Source: CAD feature listing. Evaluate the final solid. Frame: model axes, mm. A direction names the side the tool comes from. Coordinates: 2 decimals unless noted, no trailing zeros. Loops run counter-clockwise (first coordinate to the right, second up) from the corner with the lowest first, then second, coordinate; pieces in that order, holes last.
Item 1: Reachability of faces 3 (the flat face through (-10, 38, -3)), 4 (the flat face through (35, 0, -2)) from +Z, -Z, +X, -X, +Y, -Y: full face, straight path, thin tool, end or side. Return the list, or none.
Item 2: Section query B-B, the plane z = 6.5. Return the cut outline in (x, y).
Item 3: Section query C-C, the plane y = 0. Return the cut outline in (x, z).
Item 4: Pull-direction query (Z, two-part tool) for faces 1 (the flat face through (-10, -39, -3)), 2 (the cylindrical face through (-3.252, 14.643, 36.949)); classes: +Z half, -Z half, draft (parallel to the pull), parting line (faces both ways), or undercut.
Item 5: Section query A-A, the plane x = 18. Return the cut outline in (y, z).
Item 6: Line query: probe 1 along Z at (x, y) = (-19, 25); probe 2 along Y at (x, z) = (0, 38); probe 3 along Z at (x, y) = (-20.5, -10). Output: solid intervals per line, ascending.
Item 7: Pin query (flat end, axial travel): pin 1 Ø1.5 at (x, z) = (-23.5, 31.5) entering from -Y; pin 2 Ø1.5 at (y, z) = (11, -17.5) entering from +X; pin 3 Ø22.5 at (x, y) = (16, 10) entering from -Z; pin 4 Ø20 at (y, z) = (6, -5) entering from -X. Return the tip coordinate at first contact, or that it passes through.
Item 8: Section query D-D, the plane x = 0. Return the cut outline in (y, z), then the cut area to 3 significant figures.
Autodesk Inventor part; units mm, degrees
ref_plane "YZ Plane" through (0, 0, 0) normal (1, 0, 0) x (0, 1, 0)
ref_plane "XZ Plane" through (0, 0, 0) normal (0, 1, 0) x (-1, 0, 0)
ref_plane "XY Plane" through (0, 0, 0) normal (0, 0, 1) x (1, 0, 0)
sketch "Эскиз1" plane through (0, 0, 0) normal (0, 0, 1) x (1, 0, 0)
  arc A0 (45, 0) -> (-45, 0) centre (0, 0) ccw
  arc A1 (35, 0) -> (-35, 0) centre (0, 0) ccw
  line L0 (-45, 0) -> (-35, 0)
  line L1 (35, 0) -> (45, 0)
  line L2 (-63, 0) -> (63, 0)
  dimension "d0" = 45
  dimension "d1" = 35
revolve "Вращение1" add sketch "Эскиз1" angle 360 about axis through (-10, 0, 0) along (1, 0, 0) contours L1 A1 L0 A0
sketch "Эскиз2" plane through (0, 0, 0) normal (0, 0, 1) x (1, 0, 0)
  circle A0 centre (0, 0) radius 15
  dimension "d3" = 30
extrude "Выдавливание1" cut sketch "Эскиз2" along normal through all
sketch "Эскиз3" plane through (0, 0, 0) normal (0, 1, 0) x (-1, 0, 0)
  line L0 (-35, -15) -> (10, -15)
  line L1 (10, -15) -> (10, 10)
  line L2 (10, 10) -> (-35, 10)
  line L3 (-35, 10) -> (-35, -15)
  point P0 (0, 0)
  dimension "d6" = 10
  dimension "d7" = 45
  dimension "d8" = 10
  dimension "d9" = 25
extrude "Выдавливание2" cut sketch "Эскиз3" along normal through all both and the other way through all
Verdict:
1. face 3: +X, +Y, -Y
1. face 4: +Y, -Y
2. outline: (-10, -43.39) - (-10, -32.91) arc R34.39 cw to (-10, 32.91) - (-10, 43.39) arc R44.53 ccw to start; (35, -27.53) arc R44.53 ccw to (35, 27.53) - close
3. outline: (-15, 31.62) - (-15, 42.43) arc R45 ccw (long way) to (15, 42.43) - (15, 31.62) arc R35 cw to (33.54, 10) - (35, 10) - (35, -15) - (31.62, -15) arc R35 cw (long way) to start
4. face 1: undercut
4. face 2: draft
5. outline: (-40.01, 10) - (-28.3, 10) arc R30.02 cw to (28.3, 10) - (40.01, 10) arc R41.24 ccw to start; (-38.42, -15) arc R41.24 ccw to (38.42, -15) - (26, -15) arc R30.02 cw to (-26, -15) - close
6. probe 1: z = -32.23 to -15.46, 15.46 to 32.23
6. probe 2: y = -24.1 to -15, 15 to 24.1
6. probe 3: z = -38.79 to -26.55, 26.55 to 38.79
7. pin 1: stops at y = -23.21
7. pin 2: stops at x = 40.35
7. pin 3: stops at z = -44.35
7. pin 4: stops at x = -45
8. outline: (-43.87, 10) - (-33.54, 10) arc R35 cw to (-15, 31.62) - (-15, 42.43) arc R45 ccw to start; (-42.43, -15) arc R45 ccw to (42.43, -15) - (31.62, -15) arc R35 cw to (-31.62, -15) - close; (15, 31.62) arc R35 cw to (33.54, 10) - (43.87, 10) arc R45 ccw to (15, 42.43) - close
8. area: 1,700 mm2
